Can you work these out from the model? Positions are in its coordinate system, mm. Round coordinates to 2 decimals unless told otherwise and drop trailing zeros.
Q1. If I drill on line 1 (Y direction, x = -68, z = 6); line 2 (Y direction, x = 68, z = 13.45); line 3 (X direction, y = 65.5, z = 5), over which ranges is the centre line in solid material (lowest first)?
Q2. Will this pin go through, and if not, where does the flat tip stop? P1, Ø6.5, axis at x = -36, y = 105, coming from the +Z side.
Q3. If we section it at A-A (z = 12.25): Count the separate pieces of the cut face and the enclosed holes in it, plus the area to 3 significant figures.
from build123d import *

# Parameters (mm, degrees)
SKIZZE1_W                        = 180
SKIZZE1_H                        = 430
AUFSATZ_LINEAR_AUSTRAGEN1_DEPTH  = 15
SKIZZE2_R                        = 2.75
SCHNITT_LINEAR_AUSTRAGEN1_DEPTH  = 40
SKIZZE3_R                        = 3.25
SCHNITT_LINEAR_AUSTRAGEN2_DEPTH  = 40
SKIZZE6_R                        = 3.5
SCHNITT_LINEAR_AUSTRAGEN5_DEPTH  = 30
SKIZZE7_R                        = 3
SCHNITT_LINEAR_AUSTRAGEN6_DEPTH  = 40
SKIZZE8_R                        = 3
SCHNITT_LINEAR_AUSTRAGEN7_DEPTH  = 40
SKIZZE9_R                        = 5
SCHNITT_LINEAR_AUSTRAGEN8_DEPTH  = 6
SKIZZE11_R                       = 3
SCHNITT_LINEAR_AUSTRAGEN10_DEPTH = 40
SKIZZE10_R                       = 5.5
SCHNITT_LINEAR_AUSTRAGEN9_DEPTH  = 7
SKIZZE12_R                       = 2.5
SCHNITT_LINEAR_AUSTRAGEN11_DEPTH = 30


with BuildPart() as part:
    # Skizze1 → Aufsatz-Linear austragen1 (new body)
    with BuildSketch(Plane.XY):
        with Locations((0, 215)):
            Rectangle(SKIZZE1_W, SKIZZE1_H)
    extrude(amount=AUFSATZ_LINEAR_AUSTRAGEN1_DEPTH)

    # Skizze2 → Schnitt-Linear austragen1 (cut)
    with BuildSketch(Plane.XY.offset(15)):
        with Locations((36, 19)):
            Circle(SKIZZE2_R)
        with Locations((68, 19)):
            Circle(SKIZZE2_R)
        with Locations(Location((68, 55, 0), (0, 0, 180))):
            Circle(SKIZZE2_R)
        with Locations(Location((36, 55, 0), (0, 0, 180))):
            Circle(SKIZZE2_R)
        with Locations(Location((-36, 19, 0), (0, 0, 180))):
            Circle(SKIZZE2_R)
        with Locations(Location((-68, 19, 0), (0, 0, 180))):
            Circle(SKIZZE2_R)
        with Locations((-68, 55)):
            Circle(SKIZZE2_R)
        with Locations((-36, 55)):
            Circle(SKIZZE2_R)
        with Locations(Location((-36, 105, 0), (0, 0, 180))):
            Circle(SKIZZE2_R)
        with Locations(Location((-68, 105, 0), (0, 0, 180))):
            Circle(SKIZZE2_R)
        with Locations((-68, 141)):
            Circle(SKIZZE2_R)
        with Locations((-36, 141)):
            Circle(SKIZZE2_R)
        with Locations((36, 105)):
            Circle(SKIZZE2_R)
        with Locations((68, 105)):
            Circle(SKIZZE2_R)
        with Locations(Location((68, 141, 0), (0, 0, 180))):
            Circle(SKIZZE2_R)
        with Locations(Location((36, 141, 0), (0, 0, 180))):
            Circle(SKIZZE2_R)
    extrude(amount=-SCHNITT_LINEAR_AUSTRAGEN1_DEPTH, mode=Mode.SUBTRACT)

    # Skizze3 → Schnitt-Linear austragen2 (cut)
    with BuildSketch(Plane.XY.offset(15)):
        with Locations((12, 66)):
            Circle(SKIZZE3_R)
        with Locations((12, 114)):
            Circle(SKIZZE3_R)
        with Locations(Location((-12, 114, 0), (0, 0, 180))):
            Circle(SKIZZE3_R)
        with Locations(Location((-12, 66, 0), (0, 0, 180))):
            Circle(SKIZZE3_R)
    extrude(amount=-SCHNITT_LINEAR_AUSTRAGEN2_DEPTH, mode=Mode.SUBTRACT)

    # Skizze6 → Schnitt-Linear austragen5 (cut)
    with BuildSketch(Plane(origin=(0, 0, 0), x_dir=(-1, 0, 0), z_dir=(0, 0, -1))):
        with Locations((23, 395)):
            Circle(SKIZZE6_R)
        with Locations((23, 382)):
            Circle(SKIZZE6_R)
        with Locations((-23, 382)):
            Circle(SKIZZE6_R)
        with Locations((-23, 395)):
            Circle(SKIZZE6_R)
    extrude(amount=-SCHNITT_LINEAR_AUSTRAGEN5_DEPTH, mode=Mode.SUBTRACT)

    # Skizze7 → Schnitt-Linear austragen6 (cut)
    with BuildSketch(Plane.XY.offset(15)):
        with Locations((20, 415)):
            Circle(SKIZZE7_R)
        with Locations((40, 415)):
            Circle(SKIZZE7_R)
        with Locations(Location((-40, 415, 0), (0, 0, 180))):
            Circle(SKIZZE7_R)
        with Locations(Location((-20, 415, 0), (0, 0, 180))):
            Circle(SKIZZE7_R)
    extrude(amount=-SCHNITT_LINEAR_AUSTRAGEN6_DEPTH, mode=Mode.SUBTRACT)

    # Skizze8 → Schnitt-Linear austragen7 (cut)
    with BuildSketch(Plane(origin=(0, 0, 0), x_dir=(-1, 0, 0), z_dir=(0, 0, -1))):
        with Locations((22, 9)):
            Circle(SKIZZE8_R)
        with Locations((82, 9)):
            Circle(SKIZZE8_R)
        with Locations((22, 41)):
            Circle(SKIZZE8_R)
        with Locations((82, 41)):
            Circle(SKIZZE8_R)
        with Locations((-82, 41)):
            Circle(SKIZZE8_R)
        with Locations((-82, 9)):
            Circle(SKIZZE8_R)
        with Locations((-22, 9)):
            Circle(SKIZZE8_R)
        with Locations((-22, 41)):
            Circle(SKIZZE8_R)
    extrude(amount=-SCHNITT_LINEAR_AUSTRAGEN7_DEPTH, mode=Mode.SUBTRACT)

    # Skizze9 → Schnitt-Linear austragen8 (cut)
    with BuildSketch(Plane.XY.offset(15)):
        with Locations((68, 55)):
            Circle(SKIZZE9_R)
        with Locations((68, 19)):
            Circle(SKIZZE9_R)
        with Locations((36, 19)):
            Circle(SKIZZE9_R)
        with Locations((36, 55)):
            Circle(SKIZZE9_R)
        with Locations(Location((-68, 19, 0), (0, 0, 180))):
            Circle(SKIZZE9_R)
        with Locations(Location((-36, 19, 0), (0, 0, 180))):
            Circle(SKIZZE9_R)
        with Locations(Location((-68, 55, 0), (0, 0, 180))):
            Circle(SKIZZE9_R)
        with Locations(Location((-36, 55, 0), (0, 0, 180))):
            Circle(SKIZZE9_R)
        with Locations((68, 105)):
            Circle(SKIZZE9_R)
        with Locations((36, 105)):
            Circle(SKIZZE9_R)
        with Locations((-36, 105)):
            Circle(SKIZZE9_R)
        with Locations((-68, 105)):
            Circle(SKIZZE9_R)
    extrude(amount=-SCHNITT_LINEAR_AUSTRAGEN8_DEPTH, mode=Mode.SUBTRACT)

    # Skizze11 → Schnitt-Linear austragen10 (cut)
    with BuildSketch(Plane(origin=(0, 0, 0), x_dir=(-1, 0, 0), z_dir=(0, 0, -1))):
        with Locations((-52, 175)):
            Circle(SKIZZE11_R)
        with Locations((-52, 236)):
            Circle(SKIZZE11_R)
        with Locations((52, 236)):
            Circle(SKIZZE11_R)
        with Locations((52, 175)):
            Circle(SKIZZE11_R)
        with Locations((-52, 258)):
            Circle(SKIZZE11_R)
        with Locations((52, 258)):
            Circle(SKIZZE11_R)
    extrude(amount=-SCHNITT_LINEAR_AUSTRAGEN10_DEPTH, mode=Mode.SUBTRACT)

    # Skizze10 → Schnitt-Linear austragen9 (cut)
    with BuildSketch(Plane(origin=(0, 0, 0), x_dir=(-1, 0, 0), z_dir=(0, 0, -1))):
        with Locations((12, 114)):
            Circle(SKIZZE10_R)
        with Locations((-12, 114)):
            Circle(SKIZZE10_R)
        with Locations((52, 175)):
            Circle(SKIZZE10_R)
        with Locations((-52, 175)):
            Circle(SKIZZE10_R)
    extrude(amount=-SCHNITT_LINEAR_AUSTRAGEN9_DEPTH, mode=Mode.SUBTRACT)

    # Skizze12 → Schnitt-Linear austragen11 (cut)
    with BuildSketch(Plane(origin=(0, 0, 0), x_dir=(-1, 0, 0), z_dir=(0, 0, -1))):
        with Locations((82, 402)):
            Circle(SKIZZE12_R)
        with Locations((82, 158)):
            Circle(SKIZZE12_R)
        with Locations((-82, 158)):
            Circle(SKIZZE12_R)
        with Locations((-82, 402)):
            Circle(SKIZZE12_R)
    extrude(amount=-SCHNITT_LINEAR_AUSTRAGEN11_DEPTH, mode=Mode.SUBTRACT)


solid = part.part
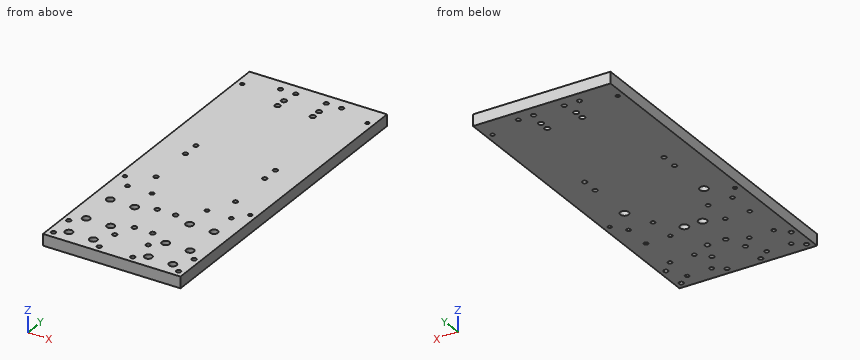
Solution:
1. line 1: y = 0 to 16.25, 21.75 to 52.25, 57.75 to 102.25, 107.75 to 138.25, 143.75 to 430
1. line 2: y = 0 to 14, 24 to 50, 60 to 100, 110 to 138.25, 143.75 to 430
1. line 3: x = -90 to -15.21, -8.79 to 8.79, 15.21 to 90
2. P1: stops at z = 9
3. separate pieces: 1
3. enclosed holes: 46
3. area: 75,500 mm2
